from build123d import *

# Parameters (mm, degrees)
BOSS_EXTRUDE1_DEPTH = 76.2
CUT_EXTRUDE1_DEPTH  = 152.364149309
SKETCH3_R           = 3.175
CUT_EXTRUDE2_DEPTH  = 152.364149309
SKETCH4_R           = 3.175
CUT_EXTRUDE3_DEPTH  = 2.524


with BuildPart() as part:
    # Sketch1 → Boss-Extrude1 (new body)
    with BuildSketch(Plane.XY):
        Polygon((0, 0), (0, 38.1), (1.524, 38.1), (1.524, -0.698546195), (-146.938943833, -128.622402846), (-153.072957039, -152.775137619), (-154.550064945, -152.4), (-148.297771302, -127.781534893), align=None)
    extrude(amount=BOSS_EXTRUDE1_DEPTH)

    # Sketch2 → Cut-Extrude1 (cut, through all)
    with BuildSketch(Plane(origin=(-108.826155859, 27.638322679, 0), x_dir=(0, 0, 1), z_dir=(-0.96923091, 0.246153293, 0))):
        Polygon((0, -185.753798063), (50.8, -185.753798063), (0, 0), align=None)
    extrude(amount=-CUT_EXTRUDE1_DEPTH, mode=Mode.SUBTRACT)

    # Sketch3 → Cut-Extrude2 (cut, through all)
    with BuildSketch(Plane(origin=(-108.826155859, 27.638322679, 0), x_dir=(0, 0, 1), z_dir=(-0.96923091, 0.246153293, 0))):
        with Locations((61.763400246, -173.053798063)):
            Circle(SKETCH3_R)
    extrude(amount=-CUT_EXTRUDE2_DEPTH, mode=Mode.SUBTRACT)

    # Sketch4 → Cut-Extrude3 (cut, through all)
    with BuildSketch(Plane.ZY):
        with Locations((19.05, 19.05)):
            Circle(SKETCH4_R)
        with Locations((57.15, 19.05)):
            Circle(SKETCH4_R)
    extrude(amount=-CUT_EXTRUDE3_DEPTH, mode=Mode.SUBTRACT)


solid = part.part
For this review, take the finished solid that the model builds, in its own axes (mm). Round coordinates to 2 decimals unless told otherwise and drop trailing zeros. Write each loop counter-clockwise with the first axis right and the second up, starting at its lowest first coordinate (ties: lowest second). Pieces come first, ordered by that corner, then holes. Notation, with made-up numbers: (46, 16) - (63, 16) arc R29 cw to (63, 38) - close; hole circle Ø7 at (29, 75). An arc over 180 degrees is marked (long way). Write item = value, one per line. Start each with the question number.
1. Consider section C-C on x = -25.5. State the section outline as (y, z) points.
2. Wall thickness on L1, parallel to Z at x = 1, y = 19; L2, parallel to X at y = 25, z = 31.5; L3, parallel to Y at x = 0.55, z = 57.15 (3 decimals): over which ranges is each line inside the solid? List them lowest first.
3. Consider section A-A on y = 19.05. State the section outline as (x, z) points (3 decimals).
4. For pin 1 Ø1.5 at (y, z) = (-120.5, 52.5) entering from +X; pin 2 Ø11.5 at (y, z) = (11.5, 54) entering from -X; pin 3 Ø1 at (x, z) = (-132.5, 53) entering from +Y; pin 4 Ø5.5 at (y, z) = (19.05, 19.05) entering from +X, all flat-tipped, find the tip position at first contact; note any pin that passes through.
5. Draft analysis for pull direction Y (two halves, no side actions). For faces 1 (the face through (0, 19, 38)), 2 (the face through (0.75, 17.12, 54.63)), 3 (the face through (-152.162, -142.998, 59.8)), state which applies: released by +Y, released by -Y, zero draft, split by the parting line, or undercut.
6. Consider section B-B on z = 19.05. State the section outline as (x, y) points (3 decimals), plus the area to 3 significant figures.
7. Consider section D-D on y = -108. State the section outline as (x, z) points.
Evaluation:
q1.outline = (-23.98, 8.07) - (-21.97, 7.54) - (-21.97, 76.2) - (-23.98, 76.2) - close
q2.L1 = 0 to 15.88, 22.22 to 53.98, 60.32 to 76.2
q2.L2 = 0 to 1.52
q2.L3 = -1.538 to 15.875, 22.225 to 38.1
q3.outline = (0, 0) - (1.524, 0) - (1.524, 15.875) - (0, 15.875) - close; (0, 22.225) - (1.524, 22.225) - (1.524, 53.975) - (0, 53.975) - close; (0, 60.325) - (1.524, 60.325) - (1.524, 76.2) - (0, 76.2) - close
q4.pin_1 = -136.64
q4.pin_2 = 0
q4.pin_3 = -113.74
q4.pin_4 = through
q5.face_1 = zero draft
q5.face_2 = undercut
q5.face_3 = released by +Y
q6.outline = (-64.421, -55.508) - (-62.617, -55.966) - (1.524, -0.699) - (1.524, 15.875) - (0, 15.875) - (0, 0) - close; (0, 22.225) - (1.524, 22.225) - (1.524, 38.1) - (0, 38.1) - close
q6.area = 178 mm2
q7.outline = (-125.34, 37.06) - (-123.01, 36.91) - (-123.01, 76.2) - (-125.34, 76.2) - close
